Check sheet for the modelled part. Datum: model origin and axes. Units: mm. A direction names the side the tool comes from. Give positions to 0.01 mm unless a question says otherwise; leave off trailing zeros. Order: outer loops, then holes, each group sorted by start corner. A loop starts at its lowest first (then second) coordinate and runs counter-clockwise, first axis right, second up. Notation, with made-up numbers: (-9.75, 21.25) -> (3.25, 21.25) arc R10 ccw to (3.25, 27.25) -> close; hole circle Ø5 at (-35.5, -16.75). An arc over 180 degrees is marked (long way). One line per question, with ' | ' between items. Start each with the question number.
from build123d import *

# Parameters (mm, degrees)
EXTRUDE_2_DEPTH     = 18
SKETCH_1_4_R        = 4
EXTRUDE_3_DEPTH     = 6
SKETCH_3_R          = 2.5
CUT_EXTRUDE_2_DEPTH = 31.6757233


with BuildPart() as part:
    # Sketch 1 → Extrude 2 (new body)
    with BuildSketch(Plane.XY):
        Polygon((8, 0), (-8, 0), (-8, -1), (-16, -1), (-16, 4), (16, 4), (16, -1), (8, -1), align=None)
    extrude(amount=EXTRUDE_2_DEPTH)

    # Sketch 1_4 → Extrude 3 (add)
    with BuildSketch(Plane.XY):
        with BuildLine():
            Line((-12, 4), (12, 4))
            Line((12, 4), (7.606095567, 17.479376982))
            ThreePointArc((7.606095567, 17.479376982), (0, 23), (-7.606095567, 17.479376982))
            Line((-7.606095567, 17.479376982), (-12, 4))
        make_face()
        with Locations((0, 15)):
            Circle(SKETCH_1_4_R, mode=Mode.SUBTRACT)
    extrude(amount=EXTRUDE_3_DEPTH)

    # Sketch 3 → Cut-Extrude 2 (cut, through all)
    with BuildSketch(Plane(origin=(0, 4, 0), x_dir=(1, 0, 0), z_dir=(0, 1, 0))):
        with Locations(Location((-12, -12, 0), (0, 0, 270))):
            Circle(SKETCH_3_R)
        with Locations(Location((12, -12, 0), (0, 0, 90))):
            Circle(SKETCH_3_R)
    extrude(amount=-CUT_EXTRUDE_2_DEPTH, mode=Mode.SUBTRACT)


solid = part.part
1. Cross-section at A-A on x = 0. Record the boundary of the cut face in (y, z), and give its area (3 significant figures).
2. Tool access check on faces 4 (the face through (14.44, 1.54, 12.54)), 5 (the face through (0, 9, 6)), 6 (the face through (-8, -0.5, 8.9)). Record the directions out of +Z, -Z, +X, -X, +Y, -Y that give a thin tool (end or side, any length) a straight path to the whole face; none if there is none.
3. Scan lines: probe 1 along X at (y, z) = (0.6, 12); probe 2 along Z at (x, y) = (12, 1.15); probe 3 along Y at (x, z) = (6.5, 10.5). Record each from-to range of solid material in increasing order.
4. Cross-section at C-C on z = 4.5. Record the boundary of the cut face in (x, y), and give its area (3 significant figures).
5. Cross-section at D-D on y = 2.5. Record the boundary of the cut face in (x, z).
6. Mould release check, pull along Y, two halves, no side actions. Record for faces 1 (the face through (0, 0, 9)), 2 (the face through (-14.44, 1.54, 11.46)), 3 (the face through (-0.521, 18.966, 2.958)): +Y half, -Y half, draft (parallel to the pull), parting line (faces both ways), or undercut.
7. Go/stop test with flat-tipped pins: pin 1 (6 mm diameter, centred on x = -12, z = 12, fed in from +Y); pin 2 (10 mm diameter, centred on x = -1.5, z = 10, fed in from -Y); pin 3 (1.5 mm diameter, centred on x = -4, y = 6, fed in from +Z). Record where each tip stops, or that it passes through.
8. Cross-section at B-B on z = 12. Record the boundary of the cut face in (x, y).
Response values:
1) outline: (0, 0) -> (11, 0) -> (11, 6) -> (4, 6) -> (4, 18) -> (0, 18) -> close; (19, 0) -> (23, 0) -> (23, 6) -> (19, 6) -> close | area: 138 mm²
2) face 4: +Y, -Y | face 5: +Z, +X, -X, +Y | face 6: +Z, -Z, -Y
3) probe 1: x = -16 to -14.5, -9.5 to 9.5, 14.5 to 16 | probe 2: z = 0 to 9.5, 14.5 to 18 | probe 3: y = 0 to 4
4) outline: (-16, -1) -> (-8, -1) -> (-8, 0) -> (8, 0) -> (8, -1) -> (16, -1) -> (16, 4) -> (12, 4) -> (7.61, 17.48) arc R8 ccw to (-7.61, 17.48) -> (-12, 4) -> (-16, 4) -> close; hole circle Ø8 at (0, 15) | area: 420 mm²
5) outline: (-16, 0) -> (16, 0) -> (16, 18) -> (-16, 18) -> close; hole circle Ø5 at (-12, 12); hole circle Ø5 at (12, 12)
6) face 1: -Y half | face 2: draft | face 3: undercut
7) pin 1: stops at y = 4 | pin 2: stops at y = 0 | pin 3: stops at z = 6
8) outline: (-16, -1) -> (-14.5, -1) -> (-14.5, 4) -> (-16, 4) -> close; (-9.5, -1) -> (-8, -1) -> (-8, 0) -> (8, 0) -> (8, -1) -> (9.5, -1) -> (9.5, 4) -> (-9.5, 4) -> close; (14.5, -1) -> (16, -1) -> (16, 4) -> (14.5, 4) -> close
